Could you check a few things on this model? Use its own coordinates, in mm. A direction names the side the tool comes from. Coordinates: 2 decimals unless noted, no trailing zeros. Order: outer loops, then holes, each group sorted by start corner. A loop starts at its lowest first (then second) coordinate and runs counter-clockwise, first axis right, second up. Notation, with made-up numbers: (89.25, 30) - (142.25, 30) arc R20 cw to (142.25, 58) - close; hole circle Ø4 at (31.5, 81). An arc over 180 degrees is marked (long way). One line per item, written item: value.
from build123d import *

# Parameters (mm, degrees)
SKETCH1_R           = 9
BOSS_EXTRUDE1_DEPTH = 6.2
CUT_EXTRUDE1_REACH  = 179.661
SKETCH2_R           = 1.5
CUT_EXTRUDE2_REACH  = 179.661
SKETCH3_R           = 3
LPATTERN1_COUNT     = 2
LPATTERN1_PITCH     = 61.2
CUT_EXTRUDE3_REACH  = 179.661
SKETCH5_W           = 95
SKETCH5_H           = 6.2


with BuildPart() as part:
    # Sketch1 → Boss-Extrude1 (new body)
    with BuildSketch(Plane(origin=(0, 0, 0), x_dir=(1, 0, 0), z_dir=(0, 1, 0))):
        with BuildLine():
            ThreePointArc((-140, 32.5), (-147.071067812, 29.571067812), (-150, 22.5))
            Line((-150, 22.5), (-150, -22.5))
            ThreePointArc((-150, -22.5), (-147.071067812, -29.571067812), (-140, -32.5))
            Line((-140, -32.5), (-105.326872165, -32.5))
            ThreePointArc((-105.326872165, -32.5), (-92.569113088, -36.000242249), (-83.383773797, -45.520833333))
            ThreePointArc((-83.383773797, -45.520833333), (8.463545381, -94.622240512), (90.138781887, -30))
            Line((90.138781887, -30), (90.138781887, 30))
            ThreePointArc((90.138781887, 30), (8.463545381, 94.622240512), (-83.383773797, 45.520833333))
            ThreePointArc((-83.383773797, 45.520833333), (-92.569113088, 36.000242249), (-105.326872165, 32.5))
            Line((-105.326872165, 32.5), (-140, 32.5))
        make_face()
        with BuildLine():
            ThreePointArc((-139, -17), (-140.5, -15.5), (-139, -14))
            Line((-139, -14), (-129, -14))
            ThreePointArc((-129, -14), (-127.5, -15.5), (-129, -17))
            Line((-129, -17), (-139, -17))
        make_face(mode=Mode.SUBTRACT)
        with BuildLine():
            ThreePointArc((-108, -17), (-109.5, -15.5), (-108, -14))
            Line((-108, -14), (-98, -14))
            ThreePointArc((-98, -14), (-96.5, -15.5), (-98, -17))
            Line((-98, -17), (-108, -17))
        make_face(mode=Mode.SUBTRACT)
        with BuildLine():
            ThreePointArc((-115, -9), (-124, 0), (-115, 9))
            Line((-115, 9), (-105, 9))
            ThreePointArc((-105, 9), (-96, 0), (-105, -9))
            Line((-105, -9), (-115, -9))
        make_face(mode=Mode.SUBTRACT)
        Circle(SKETCH1_R, mode=Mode.SUBTRACT)
        with BuildLine():
            ThreePointArc((-139, 14), (-140.5, 15.5), (-139, 17))
            Line((-139, 17), (-129, 17))
            ThreePointArc((-129, 17), (-127.5, 15.5), (-129, 14))
            Line((-129, 14), (-139, 14))
        make_face(mode=Mode.SUBTRACT)
        with BuildLine():
            ThreePointArc((-108, 14), (-109.5, 15.5), (-108, 17))
            Line((-108, 17), (-98, 17))
            ThreePointArc((-98, 17), (-96.5, 15.5), (-98, 14))
            Line((-98, 14), (-108, 14))
        make_face(mode=Mode.SUBTRACT)
    extrude(amount=-BOSS_EXTRUDE1_DEPTH)

    # Sketch2 → Cut-Extrude1 (cut, up to next)
    with BuildSketch(Plane.XZ.offset(6.2), mode=Mode.PRIVATE) as cut_extrude1_sk1:
        with Locations(Location((-7.2, 15.5, 0), (0, 0, 270))):
            Circle(SKETCH2_R)
    cut_extrude1_tool1 = extrude(cut_extrude1_sk1.sketch, amount=-CUT_EXTRUDE1_REACH, mode=Mode.PRIVATE) & part.part
    # Sketch2 → Cut-Extrude1 (cut, up to next)
    with BuildSketch(Plane.XZ.offset(6.2), mode=Mode.PRIVATE) as cut_extrude1_sk2:
        with Locations(Location((-7.2, -15.5, 0), (0, 0, 270))):
            Circle(SKETCH2_R)
    cut_extrude1_tool2 = extrude(cut_extrude1_sk2.sketch, amount=-CUT_EXTRUDE1_REACH, mode=Mode.PRIVATE) & part.part
    # Sketch2 → Cut-Extrude1 (cut, up to next)
    with BuildSketch(Plane.XZ.offset(6.2), mode=Mode.PRIVATE) as cut_extrude1_sk3:
        with Locations(Location((23.8, 15.5, 0), (0, 0, 270))):
            Circle(SKETCH2_R)
    cut_extrude1_tool3 = extrude(cut_extrude1_sk3.sketch, amount=-CUT_EXTRUDE1_REACH, mode=Mode.PRIVATE) & part.part
    # Sketch2 → Cut-Extrude1 (cut, up to next)
    with BuildSketch(Plane.XZ.offset(6.2), mode=Mode.PRIVATE) as cut_extrude1_sk4:
        with Locations(Location((23.8, -15.5, 0), (0, 0, 270))):
            Circle(SKETCH2_R)
    cut_extrude1_tool4 = extrude(cut_extrude1_sk4.sketch, amount=-CUT_EXTRUDE1_REACH, mode=Mode.PRIVATE) & part.part
    add(cut_extrude1_tool1.solids().sort_by_distance((-7.2, -6.2, 15.5))[0], mode=Mode.SUBTRACT)
    add(cut_extrude1_tool2.solids().sort_by_distance((-7.2, -6.2, -15.5))[0], mode=Mode.SUBTRACT)
    add(cut_extrude1_tool3.solids().sort_by_distance((23.8, -6.2, 15.5))[0], mode=Mode.SUBTRACT)
    add(cut_extrude1_tool4.solids().sort_by_distance((23.8, -6.2, -15.5))[0], mode=Mode.SUBTRACT)

    # Sketch3 → Cut-Extrude2 (cut, up to next)
    with BuildSketch(Plane.XZ.offset(6.2), mode=Mode.PRIVATE) as cut_extrude2_sk1:
        with Locations(Location((-56.75, -30.6, 0), (0, 0, 270))):
            Circle(SKETCH3_R)
    cut_extrude2_tool1 = extrude(cut_extrude2_sk1.sketch, amount=-CUT_EXTRUDE2_REACH, mode=Mode.PRIVATE) & part.part
    # Sketch3 → Cut-Extrude2 (cut, up to next)
    with BuildSketch(Plane.XZ.offset(6.2), mode=Mode.PRIVATE) as cut_extrude2_sk2:
        with Locations(Location((56.75, -30.6, 0), (0, 0, 270))):
            Circle(SKETCH3_R)
    cut_extrude2_tool2 = extrude(cut_extrude2_sk2.sketch, amount=-CUT_EXTRUDE2_REACH, mode=Mode.PRIVATE) & part.part
    cut_extrude2_1 = cut_extrude2_tool1.solids().sort_by_distance((-56.75, -6.2, -30.6))[0]
    add(cut_extrude2_1, mode=Mode.SUBTRACT)
    cut_extrude2_2 = cut_extrude2_tool2.solids().sort_by_distance((56.75, -6.2, -30.6))[0]
    add(cut_extrude2_2, mode=Mode.SUBTRACT)
    cut_extrude2 = cut_extrude2_1 + cut_extrude2_2  # Cut-Extrude2 as one shape, for the pattern or mirror that repeats it

    # LPattern1: Cut-Extrude2 ×2
    with Locations(*[(0, 0, i * LPATTERN1_PITCH) for i in range(1, LPATTERN1_COUNT)]):
        add(cut_extrude2, mode=Mode.SUBTRACT)

    # Sketch5 → Cut-Extrude3 (cut, up to next)
    with BuildSketch(Plane.XZ.offset(6.2), mode=Mode.PRIVATE) as cut_extrude3_sk1:
        with Locations((0, 30.6)):
            Rectangle(SKETCH5_W, SKETCH5_H)
    cut_extrude3_tool1 = extrude(cut_extrude3_sk1.sketch, amount=-CUT_EXTRUDE3_REACH, mode=Mode.PRIVATE) & part.part
    # Sketch5 → Cut-Extrude3 (cut, up to next)
    with BuildSketch(Plane.XZ.offset(6.2), mode=Mode.PRIVATE) as cut_extrude3_sk2:
        with Locations((0, -30.6)):
            Rectangle(SKETCH5_W, SKETCH5_H)
    cut_extrude3_tool2 = extrude(cut_extrude3_sk2.sketch, amount=-CUT_EXTRUDE3_REACH, mode=Mode.PRIVATE) & part.part
    add(cut_extrude3_tool1.solids().sort_by_distance((0, -6.2, 30.6))[0], mode=Mode.SUBTRACT)
    add(cut_extrude3_tool2.solids().sort_by_distance((0, -6.2, -30.6))[0], mode=Mode.SUBTRACT)


solid = part.part
Item 1: I want a section at B-B on x = -56.75. Please give me the cut outline in (y, z), then the cut area to 3 significant figures.
Conclusion:
outline: (-6.2, -76.19) - (0, -76.19) - (0, -33.6) - (-6.2, -33.6) - close; (-6.2, -27.6) - (0, -27.6) - (0, 27.6) - (-6.2, 27.6) - close; (-6.2, 33.6) - (0, 33.6) - (0, 76.19) - (-6.2, 76.19) - close
area: 870 mm²
Item 2: For faces 4 (the face through (-32, -6.2, -1)), 5 (the face through (-123, -3, 32.5)), 6 (the face through (-103, -3, -17)), which set-ups out of +Z, -Z, +X, -X, +Y, -Y let a thin tool reach every point of the face, with its end or its side?
Conclusion:
face 4: +Z, -Z, +X, -X, -Y
face 5: +Z, -X, +Y, -Y
face 6: +Y, -Y
Item 3: If I drill on probe 1 along X at (y, z) = (-2.25, 15.5); probe 2 along X at (y, z) = (-3, 0); probe 3 along Z at (x, y) = (-130.5, -1.5), over which ranges is the centre line in solid material (lowest first)?
Conclusion:
probe 1: -150 to -140.5, -127.5 to -109.5, -96.5 to -8.7, -5.7 to 22.3, 25.3 to 90.14
probe 2: -150 to -124, -96 to -9, 9 to 90.14
probe 3: -32.5 to -17, -14 to 14, 17 to 32.5
Item 4: I want a section at C-C on y = -1.5. Give the number of separate pieces and of enclosed holes in the cut face, then the cut area to 3 significant figures.
Conclusion:
separate pieces: 1
enclosed holes: 16
area: 29,700 mm²
Item 5: Thinking about a two-plate mould opening in X: for faces 1 (the face through (-134, -3, 17)), 2 (the face through (90.139, -3, 0)), 3 (the face through (9.999, -3.057, -94.472)), which applies, pulls with the +X half, pulls with the -X half, needs draft (parallel to the pull), parting line crosses it, or undercut?
Conclusion:
face 1: undercut
face 2: pulls with the +X half
face 3: parting line crosses it
Item 6: I want a section at A-A on z = 0. Please give me the cut outline in (x, y).
Conclusion:
outline: (-150, -6.2) - (-124, -6.2) - (-124, 0) - (-150, 0) - close; (-96, -6.2) - (-9, -6.2) - (-9, 0) - (-96, 0) - close; (9, -6.2) - (90.14, -6.2) - (90.14, 0) - (9, 0) - close
Item 7: I'm going to push flat-ended pins straight in: pin 1 Ø2 at (x, y) = (33, -1.5) entering from +Z; pin 2 Ø3 at (x, y) = (-108, -2.5) entering from -Z; pin 3 Ø1.5 at (x, y) = (-83, -1) entering from -Z; pin 4 Ø1.8 at (x, z) = (23.8, -15.5) entering from -Y. Where does each tip first touch, or does it pass through?
Conclusion:
pin 1: z = 89.45
pin 2: z = -32.5
pin 3: z = -47.54
pin 4: through
